Input: part model. Units: mm. Frame: model coordinates. A direction names the side the tool comes from. Give positions to 0.01 mm unless a question says otherwise; leave off trailing zeros. Order: outer loops, then holes, each group sorted by start corner. A loop starts at its lowest first (then second) coordinate and runs counter-clockwise, first axis right, second up. Notation, with made-up numbers: (10.5, -11) - (17.5, -11) arc R32 cw to (17.5, 27) - close; hole circle Ø5 at (39.25, -24.75). An arc over 180 degrees is marked (long way). Use a Markdown table: item, result.
from build123d import *

# Parameters (mm, degrees)
SKETCH001_R = 1.75
SKETCH002_W = 12
SKETCH002_H = 1


with BuildPart() as part:
    # Sketch (on XZ_Plane of Origin) → Revolution (revolve)
    with BuildSketch(Plane.XZ):
        Polygon((12.7, 0), (18, 0), (18, 7), (27.5, 7), (33.5, 2.5), (33.5, 9.5), (43.5, 9.5), (43.5, 33), (40, 33), (40, 16), (35.5, 16), (26.5, 11), (12.7, 11), align=None)
    revolve(axis=Axis((0, 0, 0), (0, 0, 1)))

    # Sketch001 (on XZ_Plane of Origin) → Revolution001 (revolve)
    with BuildSketch(Plane.XZ):
        with Locations((14.25, 5.5)):
            Circle(SKETCH001_R)
    revolve(axis=Axis((0, 0, 0), (0, 0, 1)))

    # Sketch002 (on XZ_Plane of Origin) → Groove (revolve, cut)
    with BuildSketch(Plane.XZ):
        with Locations((21, 9)):
            Rectangle(SKETCH002_W, SKETCH002_H)
    revolve(axis=Axis((0, 0, 0), (0, 0, 1)), mode=Mode.SUBTRACT)


solid = part.part
1. Mould query, pull axis Y, two halves, no side actions, for faces 6 (the face through (-8.67, -39.05, 24.38)), 7 (the face through (38, -13, 33)), 8 (the face through (-7.262, -32.703, 6.049)), 9 (the face through (-2.75, -12.4, 2.31)). Classes: pulls with the +Y half, pulls with the -Y half, needs draft (parallel to the pull), parting line crosses it, or undercut.
Response:
| item | result |
|---|---|
| face 6 | undercut |
| face 7 | needs draft |
| face 8 | parting line crosses it |
| face 9 | undercut |
2. Set-up query: faces 1 (the face through (12.3, 4.3, 0)), 2 (the face through (-14.985, 0.66, 9.007)), 3 (the face through (-2.75, -12.4, 8.62)), 4 (the face through (-22, -26, 9.5)), 5 (the face through (-5.66, 43.13, 21.41)). Return all of +Z, -Z, +X, -X, +Y, -Y with unobstructed straight access to the full face (end or side cutting, diameter ignored); none if empty.
Response:
| item | result |
|---|---|
| face 1 | -Z, +X, -X, +Y, -Y |
| face 2 | none |
| face 3 | +Z |
| face 4 | -Z |
| face 5 | +Z, -Z |
3. Pin query (flat end, axial travel): pin 1 (3 mm diameter, centred on x = 2, y = -30.5, fed in from -Z); pin 2 (4 mm diameter, centred on x = 11.5, z = 23, fed in from +Y); pin 3 (3 mm diameter, centred on y = 18, z = 16, fed in from -X). Return the tip coordinate at first contact, or that it passes through.
Response:
| item | result |
|---|---|
| pin 1 | stops at z = 3.58 |
| pin 2 | stops at y = 42.45 |
| pin 3 | stops at x = -40.25 |
4. Material intervals for line 1 along Y through (x, z) = (0, 9.1); line 2 along Z through (x, y) = (22.5, 3); line 3 along Y through (x, z) = (0, 24.75), sorted ascending.
Response:
| item | result |
|---|---|
| line 1 | y = -33.5 to -27, -15 to -12.7, 12.7 to 15, 27 to 33.5 |
| line 2 | z = 7 to 8.5, 9.5 to 11 |
| line 3 | y = -43.5 to -40, 40 to 43.5 |
5. Section query A-A (x = 0). State how many separate pieces and enclosed holes the cut face has, then the cut area to 3 significant figures.
Response:
| item | result |
|---|---|
| separate pieces | 2 |
| enclosed holes | 2 |
| area | 518 mm^2 |
6. Section query C-C (z = 20.5). Return loops of the section in (x, y).
Response:
| item | result |
|---|---|
| outline | circle Ø87 at (0, 0); hole circle Ø80 at (0, 0) |
7. Section query D-D (x = 38). Return loops of the section in (y, z), then the cut area to 3 significant figures.
Response:
| item | result |
|---|---|
| outline | (-21.17, 9.5) - (21.17, 9.5) - (21.17, 33) - (12.49, 33) - (12.49, 16) - (-12.49, 16) - (-12.49, 33) - (-21.17, 33) - close |
| area | 570 mm^2 |
